```python
from build123d import *

# Parameters (mm, degrees)
CUT_EXTRUDE1_REACH = 58.471
SKETCH5_R          = 1.25


with BuildPart() as part:
    # Sketch3 → Revolve3 (revolve)
    with BuildSketch(Plane.XY, mode=Mode.PRIVATE) as revolve3_sk:
        with BuildLine():
            Line((-23, 0), (0, 0))
            Line((0, 0), (0, 3))
            Line((0, 3), (-19.171572875, 3))
            ThreePointArc((-19.171572875, 3), (-19.93693974, 3.152240935), (-20.585786438, 3.585786438))
            Line((-20.585786438, 3.585786438), (-25, 8))
            Line((-25, 8), (-25, 1))
            ThreePointArc((-25, 1), (-24.707106781, 0.292893219), (-24, 0))
            Line((-24, 0), (-23, 0))
        make_face()
    revolve(revolve3_sk.sketch.rotate(Axis((0, 0, 0), (0, 1, 0)), 270), axis=Axis((0, 0, 0), (0, 1, 0)))

    # Sketch5 → Cut-Extrude1 (cut, up to next)
    with BuildSketch(Plane.XY.offset(25), mode=Mode.PRIVATE) as cut_extrude1_sk1:
        with Locations((-2, 4.5)):
            Circle(SKETCH5_R)
    cut_extrude1_tool1 = extrude(cut_extrude1_sk1.sketch, amount=-CUT_EXTRUDE1_REACH, mode=Mode.PRIVATE) & part.part
    # Sketch5 → Cut-Extrude1 (cut, up to next)
    with BuildSketch(Plane.XY.offset(25), mode=Mode.PRIVATE) as cut_extrude1_sk2:
        with Locations((2, 4.5)):
            Circle(SKETCH5_R)
    cut_extrude1_tool2 = extrude(cut_extrude1_sk2.sketch, amount=-CUT_EXTRUDE1_REACH, mode=Mode.PRIVATE) & part.part
    add(cut_extrude1_tool1.solids().sort_by_distance((-2, 4.5, 25))[0], mode=Mode.SUBTRACT)
    add(cut_extrude1_tool2.solids().sort_by_distance((2, 4.5, 25))[0], mode=Mode.SUBTRACT)


solid = part.part
```
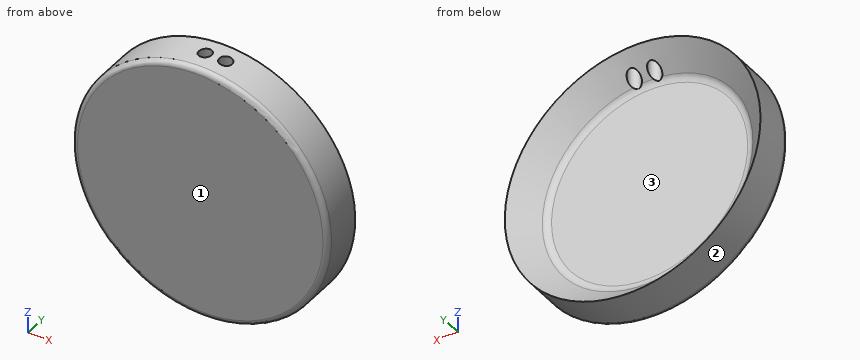
Part model, mm, in its own coordinate system. Face numbers are marked on the shaded views. Round coordinates to 2 decimals unless told otherwise and drop trailing zeros. Write each loop counter-clockwise with the first axis right and the second up, starting at its lowest first coordinate (ties: lowest second). Pieces come first, ordered by that corner, then holes. Notation, with made-up numbers: (48.25, 6.5) -> (80.25, 6.5) arc R18 cw to (80.25, 32.5) -> close; hole circle Ø8 at (77, 7.5). An arc over 180 degrees is marked (long way). Return JSON: item names as keys, results as strings. Group by question number.
Q1. Mould opens along X. For the marked faces 1, 2 and 3 say: pulls with the +X half, pulls with the -X half, needs draft (parallel to the pull), parting line crosses it, or undercut.
Q2. Saw through at A-A on x = 0. Write the cut outline in (y, z).
Q3. Saw through at B-B on y = 4.5. Write the cut outline in (x, z), plus the area to 3 significant figures.
Q4. Probe L1, parallel to X at y = 0.5, z = 6.5; L2, parallel to X at y = 3.5, z = -3.5; L3, parallel to Y at x = 14, z = -4. List the from-to ranges inside material, lowest first. Write a range as [from, to].
Q5. Saw through at C-C on y = 7. Write the cut outline in (x, z), plus the area to 3 significant figures.
Q6. Pin check, flat tips, straight feed: pin 1 (1.5 mm diameter, centred on x = 2, y = 5.5, fed in from -Z); pin 2 (2 mm diameter, centred on x = 19, z = 8, fed in from +Y); pin 3 (2 mm diameter, centred on x = 2, y = 4.5, fed in from +Z). Stop position of each tip, or through.
Answer:
{
 "1": {"face 1": "needs draft", "face 2": "parting line crosses it", "face 3": "undercut"},
 "2": {"outline": "(0, -24) arc R1 ccw to (1, -25) -> (8, -25) -> (3.59, -20.59) arc R2 cw to (3, -19.17) -> (3, 19.17) arc R2 cw to (3.59, 20.59) -> (8, 25) -> (1, 25) arc R1 ccw to (0, 24) -> close"},
 "3": {"outline": "(-3.25, 21.25) -> (-3.25, 24.79) arc R25 ccw (long way) to (3.25, 24.79) -> (3.25, 21.25) arc R21.5 cw (long way) to start; (-0.75, 21.49) arc R21.5 cw to (0.75, 21.49) -> (0.75, 24.99) arc R25 ccw to (-0.75, 24.99) -> close", "area": "494 mm2"},
 "4": {"L1": "[-24, 24]", "L2": "[-24.75, -20.19], [20.19, 24.75]", "L3": "[0, 3]"},
 "5": {"outline": "circle Ø50 at (0, 0); hole circle Ø48 at (0, 0)", "area": "154 mm2"},
 "6": {"pin 1": "z = -24.97", "pin 2": "y = 4.62", "pin 3": "z = -20.39"}
}
